Verification items for the finished model (mm, model axes). Coordinates: 2 decimals unless noted, no trailing zeros. Order: outer loops, then holes, each group sorted by start corner. A loop starts at its lowest first (then second) coordinate and runs counter-clockwise, first axis right, second up. Notation, with made-up numbers: (2.5, 20) -> (15.5, 20) arc R19 ccw to (15.5, 42) -> close; hole circle Ø3 at (-1.75, -14). An arc over 180 degrees is marked (long way). Write item = value, one per line. Start each with the question number.
from build123d import *

# Parameters (mm, degrees)
F0_R     = 1.5
F1_DEPTH = 1.5


with BuildPart() as f1:
    # F0 (on Top) → F1 (new body)
    with BuildSketch(Plane.XY):
        with BuildLine():
            Line((0, 17), (0, 5))
            ThreePointArc((0, 5), (1.464466, 1.464466), (5, 0))
            Line((5, 0), (25, 0))
            ThreePointArc((25, 0), (29.818575, 3.665332), (27.572479, 9.287465))
            Line((27.572479, 9.287465), (7.572479, 21.287465))
            ThreePointArc((7.572479, 21.287465), (2.536506, 21.351), (0, 17))
        make_face()
        with Locations((5, 5)):
            Circle(F0_R, mode=Mode.SUBTRACT)
        with Locations((25, 5)):
            Circle(F0_R, mode=Mode.SUBTRACT)
        with Locations((5, 17)):
            Circle(F0_R, mode=Mode.SUBTRACT)
    extrude(amount=F1_DEPTH)


solid = f1.part
Item 1: Section check C-C (x = 6). Record the boundary of the cut face in (y, z).
Item 2: Section check D-D (x = 10.5). Record the boundary of the cut face in (y, z), then the cut area to 3 significant figures.
Item 3: Section check B-B (y = 4.25). Record the boundary of the cut face in (x, z), then the cut area to 3 significant figures.
Item 4: Mould release check, pull along Y, two halves, no side actions. Record for faces 1 (the flat face through (11, 9, 0)), 2 (the cylindrical face through (4.805, 18.487, 0.74)), 3 (the cylindrical face through (23.5, 5.07, 0.74)), 4 (the flat face through (17.712, 15.203, 0.74)): pulls with the +Y half, pulls with the -Y half, needs draft (parallel to the pull), parting line crosses it, or undercut.
Item 5: Section check A-A (z = 0.85). Record the boundary of the cut face in (x, y).
Item 6: Thickness scan on line 1 (Y direction, x = 5, z = 0.55); line 2 (Y direction, x = 6, z = 1.2); line 3 (Y direction, x = 3, z = 0.65). Record the ranges inside material, lowest first.
Filled sheet:
q1.outline = (0, 0) -> (3.88, 0) -> (3.88, 1.5) -> (0, 1.5) -> close; (6.12, 0) -> (15.88, 0) -> (15.88, 1.5) -> (6.12, 1.5) -> close; (18.12, 0) -> (21.9, 0) -> (21.9, 1.5) -> (18.12, 1.5) -> close
q2.outline = (0, 0) -> (19.53, 0) -> (19.53, 1.5) -> (0, 1.5) -> close
q2.area = 29.3 mm^2
q3.outline = (0.06, 0) -> (3.7, 0) -> (3.7, 1.5) -> (0.06, 1.5) -> close; (6.3, 0) -> (23.7, 0) -> (23.7, 1.5) -> (6.3, 1.5) -> close; (26.3, 0) -> (29.94, 0) -> (29.94, 1.5) -> (26.3, 1.5) -> close
q3.area = 37.0 mm^2
q4.face_1 = needs draft
q4.face_2 = undercut
q4.face_3 = undercut
q4.face_4 = pulls with the +Y half
q5.outline = (0, 5) arc R5 ccw to (5, 0) -> (25, 0) arc R5 ccw to (27.57, 9.29) -> (7.57, 21.29) arc R5 ccw to (0, 17) -> close; hole circle Ø3 at (5, 5); hole circle Ø3 at (5, 17); hole circle Ø3 at (25, 5)
q6.line_1 = 0 to 3.5, 6.5 to 15.5, 18.5 to 22
q6.line_2 = 0 to 3.88, 6.12 to 15.88, 18.12 to 21.9
q6.line_3 = 0.42 to 21.58
